Build history of the part. All positions in model axes, mm. Face numbers are marked on the shaded views. A direction names the side the tool comes from. Give positions to 0.01 mm unless a question says otherwise; leave off trailing zeros. Order: outer loops, then holes, each group sorted by start corner. A loop starts at its lowest first (then second) coordinate and runs counter-clockwise, first axis right, second up. Notation, with made-up numbers: (4.25, -21.5) -> (43.25, -21.5) arc R13 ccw to (43.25, -2.5) -> close; hole circle Ø7 at (43.5, 35). An arc over 180 degrees is marked (long way). One line per question, with ' | ' between items. Start each with the question number.
(1) Which spindle directions (+Z, -Z, +X, -X, +Y, -Y) get a long thin tool onto all of the face, cutting with end or side? Do the marked faces 1, 2 and 3. Say none if no direction does.
(2) Cut at B-B (y = -0.5). Give the cut face in (x, z).
(3) Cut at A-A (x = -7.5). Give the cut face in (y, z).
(4) Pull direction Y, two halves, no side cores. Call the marked faces 4, 5 and 6: +Y half, -Y half, draft (parallel to the pull), parting line (faces both ways), or undercut.
(5) Pin check, flat tip, straight feed: pin 1 Ø7.5 at (y, z) = (4, 12.5) entering from -X. Stop position of the tip, or through.
(6) Drill centre lines: L1, parallel to Y at x = -8.5, z = 18; L2, parallel to X at y = 0, z = 14.5; L3, parallel to X at y = 12.5, z = 12.25. Where is each one in solid material? Low to high. Write a range as from..to.
(7) Cut at D-D (z = 4). Give the cut face in (x, y), then the cut area to 3 significant figures.
(8) Cut at C-C (z = 13). Give the cut face in (x, y), then the cut area to 3 significant figures.
from build123d import *

# Parameters (mm, degrees)
F1_DEPTH    = 23
F2_W        = 3.6
F2_H        = 13.6
F3_DEPTH    = 48.7
F4_T1_DEPTH = 32.5
F5_R        = 3


# Not quite as in the source:
# - a fillet or chamfer that OpenCascade refuses, or shapes differently, is made with other operations: its cross-section is extruded or revolved along the edge and cut away or added


with BuildPart() as f1:
    # F0 (on Top) → F1 (new body)
    with BuildSketch(Plane.XY):
        Polygon((12.7659387215, -17.2428843321), (12.7659387215, 15.2571156679), (-26.2254474751, 15.2571156679), (-26.2254474751, 10.2571156679), (-0.2340612785, 10.2571156679), (-0.2340612785, -12.2428843321), (-26.2254474751, -12.2428843321), (-26.2254474751, -17.2428843321), align=None)
    extrude(amount=F1_DEPTH)

    # F2 (on face) → F3 (cut)
    with BuildSketch(Plane.XZ.offset(17.2428843321)):
        with Locations((6.5272997685, 11.6975279525)):
            Rectangle(F2_W, F2_H)
    extrude(amount=-F3_DEPTH, mode=Mode.SUBTRACT)

    # F4: fillet of radius 2 on 4 edges, made by hand

    # F4_s2 → F4_t1 (join)
    with BuildSketch(Plane.XZ.offset(-15.2571156679)):
        with BuildLine():
            ThreePointArc((4.7272997685, 16.4975279525), (5.3130862061, 17.9117415149), (6.7272997685, 18.4975279525))
            Line((6.7272997685, 18.4975279525), (4.7272997685, 18.4975279525))
            Line((4.7272997685, 18.4975279525), (4.7272997685, 16.4975279525))
        make_face()
        with BuildLine():
            ThreePointArc((4.7272997685, 6.8975279525), (5.3130862061, 5.4833143901), (6.7272997685, 4.8975279525))
            Line((6.7272997685, 4.8975279525), (4.7272997685, 4.8975279525))
            Line((4.7272997685, 4.8975279525), (4.7272997685, 6.8975279525))
        make_face()
        with BuildLine():
            ThreePointArc((6.3272997685, 18.4975279525), (7.7415133308, 17.9117415149), (8.3272997685, 16.4975279525))
            Line((8.3272997685, 16.4975279525), (8.3272997685, 18.4975279525))
            Line((8.3272997685, 18.4975279525), (6.3272997685, 18.4975279525))
        make_face()
        with BuildLine():
            ThreePointArc((8.3272997685, 6.8975279525), (7.7415133308, 5.4833143901), (6.3272997685, 4.8975279525))
            Line((6.3272997685, 4.8975279525), (8.3272997685, 4.8975279525))
            Line((8.3272997685, 4.8975279525), (8.3272997685, 6.8975279525))
        make_face()
    extrude(amount=F4_T1_DEPTH)

    # F5
    f5_edges = [f1.edges().sort_by_distance(p)[0] for p in [
        (-6.729754, 15.257116, 0),
        (-26.225447, 15.257116, 11.5),
        (-6.729754, 15.257116, 23),
        (-6.729754, -17.242884, 23),
        (12.765939, -0.992884, 23),
        (-6.729754, -17.242884, 0),
        (12.765939, -0.992884, 0),
        (12.765939, -17.242884, 11.5),
        (12.765939, 15.257116, 11.5),
        (-26.225447, -17.242884, 11.5),
    ]]
    fillet(f5_edges, radius=F5_R)


solid = f1.part
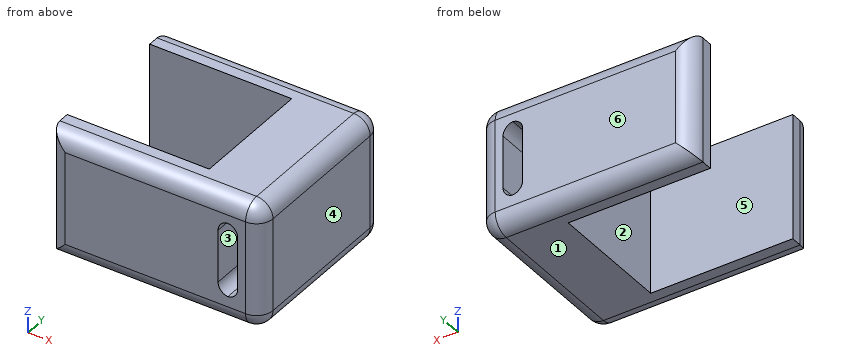
Result set:
1) face 1: -Z, +X, -X, +Y, -Y | face 2: +Z, -Z, -X | face 3: +Y, -Y
2) outline: (-0.23, 0) -> (9.77, 0) arc R3 ccw to (12.77, 3) -> (12.77, 20) arc R3 ccw to (9.77, 23) -> (-0.23, 23) -> close; hole (4.73, 6.9) arc R2 ccw to (6.53, 4.91) arc R2 ccw to (8.33, 6.9) -> (8.33, 16.5) arc R2 ccw to (6.53, 18.49) arc R2 ccw to (4.73, 16.5) -> close
3) outline: (-17.24, 3) arc R3 ccw to (-14.24, 0) -> (-12.24, 0) -> (-12.24, 23) -> (-14.24, 23) arc R3 ccw to (-17.24, 20) -> close; (10.26, 0) -> (12.26, 0) arc R3 ccw to (15.26, 3) -> (15.26, 20) arc R3 ccw to (12.26, 23) -> (10.26, 23) -> close
4) face 4: draft | face 5: undercut | face 6: +Y half
5) pin 1: stops at x = -0.23
6) L1: y = -17.24..-12.24, 10.26..15.26 | L2: x = -0.23..4.73, 8.33..12.77 | L3: x = -26.22..4.73, 8.33..12.76
7) outline: (-26.23, -14.24) arc R3 ccw to (-23.23, -17.24) -> (9.77, -17.24) arc R3 ccw to (12.77, -14.24) -> (12.77, 12.26) arc R3 ccw to (9.77, 15.26) -> (-23.23, 15.26) arc R3 ccw to (-26.23, 12.26) -> (-26.23, 10.26) -> (-0.23, 10.26) -> (-0.23, -12.24) -> (-26.23, -12.24) -> close | area: 675 mm2
8) outline: (-26.23, -14.24) arc R3 ccw to (-23.23, -17.24) -> (4.73, -17.24) -> (4.73, 15.26) -> (-23.23, 15.26) arc R3 ccw to (-26.23, 12.26) -> (-26.23, 10.26) -> (-0.23, 10.26) -> (-0.23, -12.24) -> (-26.23, -12.24) -> close; (8.33, -17.24) -> (9.77, -17.24) arc R3 ccw to (12.77, -14.24) -> (12.77, 12.26) arc R3 ccw to (9.77, 15.26) -> (8.33, 15.26) -> close | area: 558 mm2
